Autodesk Inventor part; units mm, degrees
ref_plane "YZ Plane" through (0, 0, 0) normal (1, 0, 0) x (0, 1, 0)
ref_plane "XZ Plane" through (0, 0, 0) normal (0, 1, 0) x (-1, 0, 0)
ref_plane "XY Plane" through (0, 0, 0) normal (0, 0, 1) x (1, 0, 0)
sketch "Sketch1" plane through (0, 0, 0) normal (0, 0, 1) x (1, 0, 0)
  line L0 (-2.5, 15) -> (2.5, 15)
  line L1 (7.5, 10) -> (7.5, -15)
  line L2 (7.5, -15) -> (-7.5, -15)
  line L3 (-7.5, -15) -> (-7.5, 10)
  line L4 (-7.5, 15) -> (7.5, -15) construction
  line L5 (7.5, 15) -> (-7.5, -15) construction
  arc A0 (-2.5, 15) -> (-7.5, 10) centre (-2.5, 10) ccw
  arc A1 (7.5, 10) -> (2.5, 15) centre (2.5, 10) ccw
  circle A2 centre (0, 10) radius 1.5
  point P0 (0, 0)
  dimension "d0" = 15
  dimension "HOOK_LEN" = 30
  dimension "d2" = 5
  dimension "d3" = 3
  dimension "d13" = 5
extrude "Extrusion1" add sketch "Sketch1" along normal blind 5
sketch "Sketch2" plane through (0, 0, 5) normal (0, 0, 1) x (1, 0, 0)
  circle A0 centre (0, 10) radius 1.5
  point P0 (0, 0)
  point P1 (0, 10)
hole "Hole1" at (0, 10, 5) direction (0, 0, -1) diameter 4 end through all countersink diameter 6 countersink angle 90
sketch "Sketch3" plane through (-7.5, -15, 0) normal (-1, 0, 0) x (0, 0, 1)
  line L0 (5, 0) -> (15, 0)
  arc A0 (15, 0) -> (20, 5) centre (15, 5) ccw
  line L1 (20, 5) -> (20, 15)
  line L2 (20, 15) -> (20, 5)
  arc A1 (15, 3) -> (17, 5) centre (15, 5) ccw
  line L3 (15, 3) -> (7, 3)
  line L4 (17, 5) -> (17, 15)
  arc A2 (20, 15) -> (17, 15) centre (18.5, 15) ccw
  arc A3 (5, 5) -> (7, 3) centre (7, 5) ccw
  line L5 (5, 25) -> (5, 0)
  line L6 (5, 5) -> (5, 0)
  point P0 (0, 15)
  dimension "d14" = 10
  dimension "d15" = 10
  dimension "d17" = 3
  dimension "d19" = 4
extrude "Extrusion2" add sketch "Sketch3" against normal up to surface (15 mm away)
sketch "Sketch4" plane through (-7.5, -15, 0) normal (-1, 0, 0) x (0, 0, 1)
  arc A0 (0, 2) -> (2, 0) centre (2, 2) ccw
  line L0 (0, 25) -> (0, 0)
  line L1 (0, 0) -> (15, 0)
  point P0 (0, 15)
  dimension "d22" = 4
extrude "Extrusion3" cut sketch "Sketch4" against normal through all
fillet "Fillet1" radius 1 28 edges at (7.5, -11.4142, 5.5858) (7.5, 0, 5) (6.0355, 13.5355, 5) (0, 15, 5) (-6.0355, 13.5355, 5) (-7.5, 0, 5) (-7.5, -11.4142, 5.5858) (-7.5, -12, 11) (-7.5, -11.4142, 16.4142) (-7.5, -5, 17) (-7.5, 1.5, 18.5) (-7.5, -5, 20) (-7.5, -13.5355, 18.5355) (-7.5, -15, 8.5) (-7.5, -14.4142, 0.5858) (-7.5, -1.5, 0) (-6.0355, 13.5355, 0) (0, 15, 0) (6.0355, 13.5355, 0) (7.5, -1.5, 0) (7.5, -14.4142, 0.5858) (7.5, -15, 8.5) (7.5, -13.5355, 18.5355) (7.5, -5, 20) (7.5, 1.5, 18.5) (7.5, -5, 17) (7.5, -11.4142, 16.4142) (7.5, -12, 11)
properties part number "hook_straight"
Geometry check sheet. Reference: the model listing, model coordinates, mm. A direction names the side the tool comes from. Round coordinates to 2 decimals unless told otherwise and drop trailing zeros. Write each loop counter-clockwise with the first axis right and the second up, starting at its lowest first coordinate (ties: lowest second). Pieces come first, ordered by that corner, then holes. Notation, with made-up numbers: (43, 42.25) -> (77, 42.25) arc R23 ccw to (77, 50.25) -> close; hole circle Ø2 at (-27, 70). An arc over 180 degrees is marked (long way). Put each result on its own line as item: value.
1) Cross-section at B-B, the plane z = 10.25. Enter the section's corners in (x, y).
Recorded:
outline: (-7.5, -14) arc R1 ccw to (-6.5, -15) -> (6.5, -15) arc R1 ccw to (7.5, -14) -> (7.5, -13) arc R1 ccw to (6.5, -12) -> (-6.5, -12) arc R1 ccw to (-7.5, -13) -> close
2) Thickness scan on probe 1 along X at (y, z) = (10, 1.1); probe 2 along Z at (x, y) = (-1.75, -4.5); probe 3 along Y at (x, z) = (0, 2.6). Record the ranges inside material, lowest first. Write a range as from..to.
Recorded:
probe 1: x = -7.5..-2, 2..7.5
probe 2: z = 0..5, 17..20
probe 3: y = -15..8, 12..15
3) Release check for a two-part mould opening along Z. For faces 1 (the face through (0, -14, 18)), 2 (the face through (7.215, -0.14, 4.699)), 3 (the face through (7.215, -14.699, 8.409)) record: pulls with the +Z half, pulls with the -Z half, needs draft (parallel to the pull), parting line crosses it, or undercut.
Recorded:
face 1: pulls with the +Z half
face 2: undercut
face 3: needs draft
4) Depth check by flat-ended pin: P1, Ø5, axis at x = 2.5, z = 7, coming from the +Y side; P2, Ø6.5, axis at x = 0, y = 10, coming from the +Z side; P3, Ø1.5, axis at y = -10, z = 17, coming from the -X side. Enter the tip coordinate at first touch or a pass-through.
Recorded:
P1: stops at y = 14.87
P2: stops at z = 5
P3: stops at x = -7.47
5) Access from +Z, -Z, +X, -X, +Y, -Y to the whole of each face (thin tool, end or side, straight path). Record for faces 4 (the face through (0, -5, 17)), 5 (the face through (7.215, -4.93, 17.301)), 6 (the face through (0, -5, 20)), 7 (the face through (-7.215, -12.301, 10.944)).
Recorded:
face 4: +X, -X, +Y
face 5: +X, +Y
face 6: +Z, +X, -X, +Y, -Y
face 7: -X, +Y
6) Cross-section at A-A, the plane x = 0. Enter the section's corners in (y, z), plus the area to 3 significant figures.
Recorded:
outline: (-15, 2) arc R2 ccw to (-13, 0) -> (8, 0) -> (8, 4) -> (7, 5) -> (-10, 5) arc R2 cw to (-12, 7) -> (-12, 15) arc R2 cw to (-10, 17) -> (0, 17) arc R1.5 ccw to (0, 20) -> (-10, 20) arc R5 ccw to (-15, 15) -> close; (12, 0) -> (14, 0) arc R1 ccw to (15, 1) -> (15, 4) arc R1 ccw to (14, 5) -> (13, 5) -> (12, 4) -> close
area: 209 mm2
7) Cross-section at C-C, the plane y = 2.5. Enter the section's corners in (x, z).
Recorded:
outline: (-7.5, 1) arc R1 ccw to (-6.5, 0) -> (6.5, 0) arc R1 ccw to (7.5, 1) -> (7.5, 4) arc R1 ccw to (6.5, 5) -> (-6.5, 5) arc R1 ccw to (-7.5, 4) -> close
